Geometry check sheet. Reference: drawing and pictorial views, mm from the part's lowest x, y, z. A direction names the side the tool comes from. Round coordinates to 2 decimals unless told otherwise and drop trailing zeros. Order: outer loops, then holes, each group sorted by start corner. A loop starts at its lowest first (then second) coordinate and runs counter-clockwise, first axis right, second up.
Q1. Set-up check for the marked faces 1 and 2: record each of +Z, -Z, +X, -X, +Y, -Y from which the full face is reachable in a straight line by a thin tool's end or side.
Q2. Depth check by flat-ended pin: P1, Ø4, axis at x = 10, y = 10, coming from the -Z side; P2, Ø8, axis at x = 23.5, z = 13.5, coming from the +Y side; P3, Ø8, axis at x = 23.5, z = 25.5, coming from the -Y side; P4, Ø4, axis at y = 6.5, z = 9, coming from the +X side. Enter the tip coordinate at first touch or a pass-through.
Q3. Mould release check, pull along Z, two halves, no side actions. Record for the marked faces 3, 4, 5 and 6: +Z half, -Z half, draft (parallel to the pull), parting line (faces both ways), or undercut.
Q4. Cross-section at B-B on z = 25. Record the cut outline in (x, y), then the cut area to 3 significant figures.
Q5. Scan lines: probe 1 along Y at (x, z) = (22, 5.5); probe 2 along Z at (x, y) = (26, 5.5); probe 3 along Z at (x, y) = (7.5, 9). Record each from-to range of solid material in increasing order.
Q6. Cross-section at D-D on z = 29. Record the cut outline in (x, y), then the cut area to 3 significant figures.
Q7. Cross-section at A-A on y = 2.5. Record the cut outline in (x, z) (1 decimal).
Q8. Cross-section at C-C on x = 8.5. Record the cut outline in (y, z) (1 decimal), then the cut area to 3 significant figures.
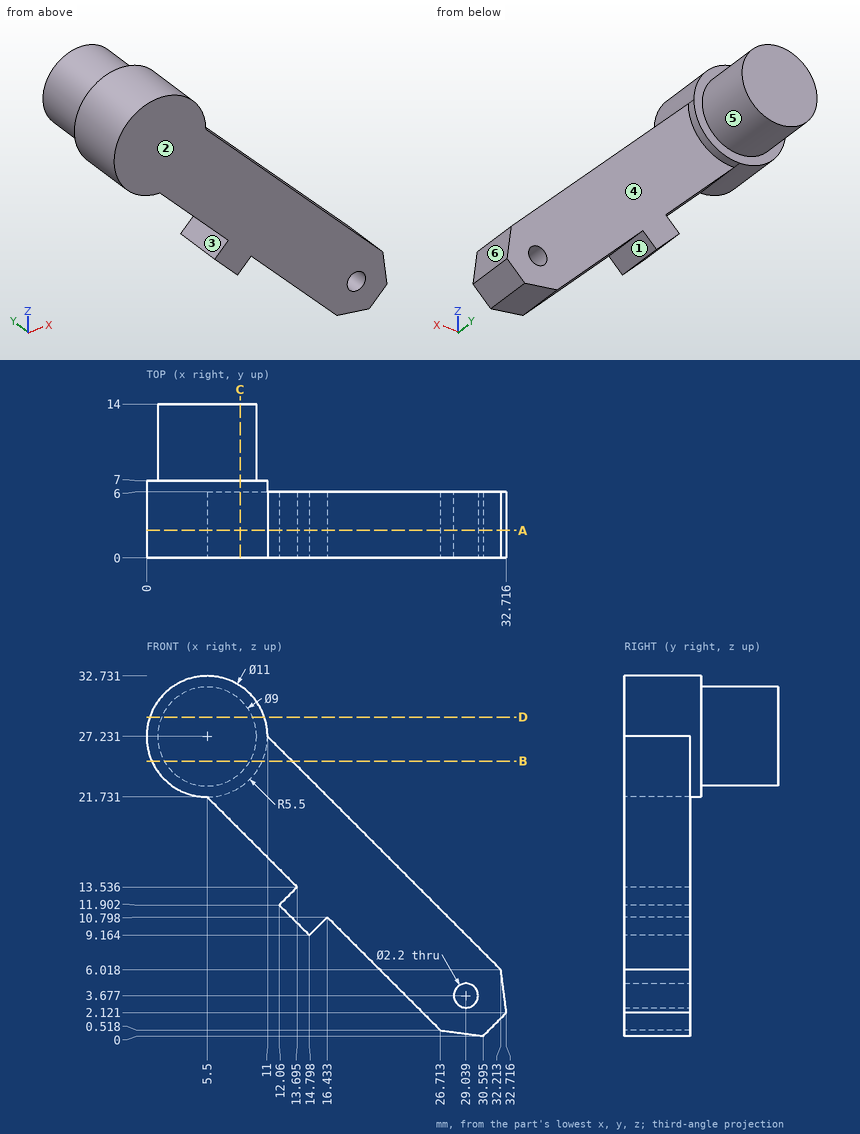
Results found:
1. face 1: -Z, +Y, -Y
1. face 2: +Z, -Z, +X, -X, -Y
2. P1: stops at z = 23.49
2. P2: stops at y = 6
2. P3: passes through
2. P4: stops at x = 31.17
3. face 3: undercut
3. face 4: draft
3. face 5: parting line
3. face 6: +Z half
4. outline: (0.47, 0) - (13.23, 0) - (13.23, 6) - (10.53, 6) - (10.53, 7) - (9.41, 7) - (9.41, 14) - (1.59, 14) - (1.59, 7) - (0.47, 7) - close
4. area: 141 mm2
5. probe 1: y = 0 to 6
5. probe 2: z = 1.23 to 12.23
5. probe 3: z = 23.2 to 31.26
6. outline: (0.29, 0) - (10.71, 0) - (10.71, 7) - (9.64, 7) - (9.64, 14) - (1.36, 14) - (1.36, 7) - (0.29, 7) - close
6. area: 131 mm2
7. outline: (5.5, 21.7) - (13.7, 13.5) - (12.1, 11.9) - (14.8, 9.2) - (16.4, 10.8) - (26.7, 0.5) - (30.6, 0) - (32.7, 2.1) - (32.2, 6) - (11, 27.2) arc R5.5 ccw (long way) to start; hole circle Ø2.2 at (29, 3.7)
8. outline: (0, 18.7) - (6, 18.7) - (6, 22.6) - (7, 22.6) - (7, 23.9) - (14, 23.9) - (14, 30.6) - (7, 30.6) - (7, 31.8) - (0, 31.8) - close
8. area: 135 mm2
